For this review, use the dimensioned drawing (mm, ordinates from the lowest corner) and the shaded views. Give positions to 0.01 mm unless a question says otherwise; leave off trailing zeros. Order: outer loops, then holes, each group sorted by start corner. A loop starts at its lowest first (then second) coordinate and runs counter-clockwise, first axis right, second up.
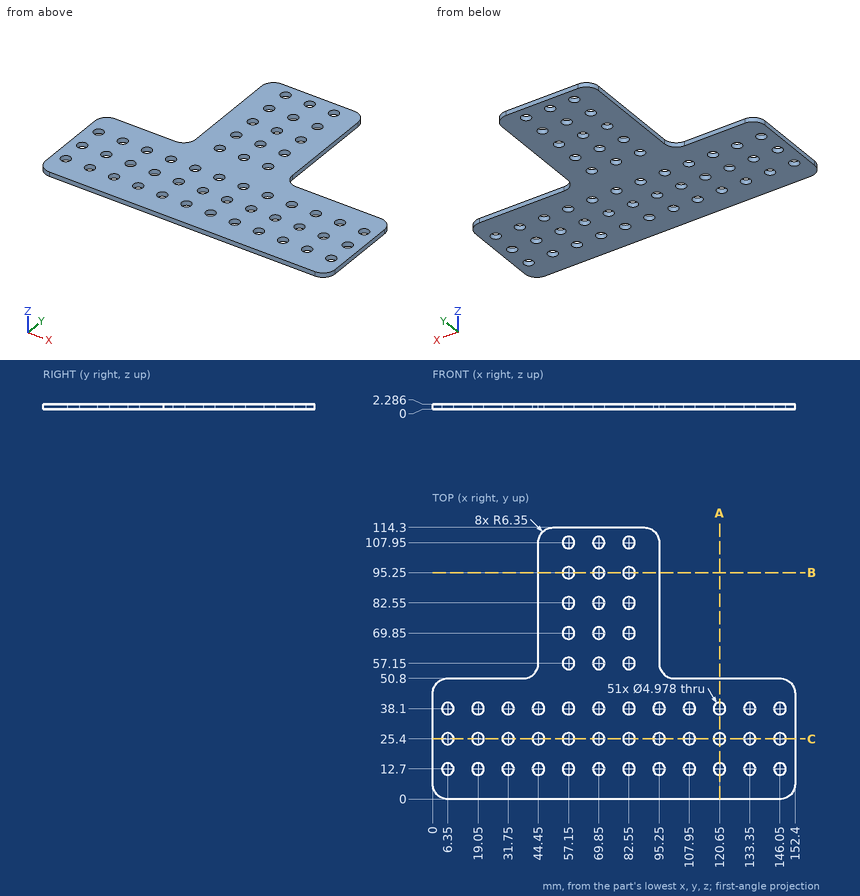
1. Insertion check: pin 1 (1 mm diameter, centred on y = 79, z = 1.5, fed in from +X). The pin has a flat end and moves straight along its axis. Give the tip position at first contact, or say it passes through.
2. Take a section at C-C (y = 25.4). Count the separate pieces of the cut face and the enclosed holes in it, and give its area (3 significant figures).
3. To check wall thickness, follow line 1 (Y direction, x = 121, z = 1.7) (1 decimal); line 2 (Y direction, x = 146.5, z = 1.1) (1 decimal); line 3 (Y direction, x = 89, z = 1.65). State the ranges of each line that lie inside material, in increasing order.
4. Take a section at A-A (x = 120.65). Write out the cut boundary in (y, z).
5. Take a section at B-B (y = 95.25). Write out the cut boundary in (x, z).
Answer:
1. pin 1: stops at x = 95.25
2. separate pieces: 13
2. enclosed holes: 0
2. area: 212 mm2
3. line 1: y = 0 to 10.2, 15.2 to 22.9, 27.9 to 35.6, 40.6 to 50.8
3. line 2: y = 0 to 10.3, 15.1 to 23, 27.8 to 35.7, 40.5 to 50.8
3. line 3: y = 0 to 114.3
4. outline: (0, 0) - (10.21, 0) - (10.21, 2.29) - (0, 2.29) - close; (15.19, 0) - (22.91, 0) - (22.91, 2.29) - (15.19, 2.29) - close; (27.89, 0) - (35.61, 0) - (35.61, 2.29) - (27.89, 2.29) - close; (40.59, 0) - (50.8, 0) - (50.8, 2.29) - (40.59, 2.29) - close
5. outline: (44.45, 0) - (54.66, 0) - (54.66, 2.29) - (44.45, 2.29) - close; (59.64, 0) - (67.36, 0) - (67.36, 2.29) - (59.64, 2.29) - close; (72.34, 0) - (80.06, 0) - (80.06, 2.29) - (72.34, 2.29) - close; (85.04, 0) - (95.25, 0) - (95.25, 2.29) - (85.04, 2.29) - close
